Verification items for the finished model (mm, model axes). A direction names the side the tool comes from. Round coordinates to 2 decimals unless told otherwise and drop trailing zeros. Order: outer loops, then holes, each group sorted by start corner. A loop starts at its lowest first (then second) coordinate and runs counter-clockwise, first axis right, second up. Notation, with made-up numbers: (-6, 21.25) -> (31, 21.25) arc R16 cw to (31, 46.25) -> close; hole circle Ø9 at (15.5, 60.25). An arc over 180 degrees is marked (long way). Return JSON: item names as keys, results as strings. Group by question number.
1) Draft check along Y on faces 1 (the cylindrical face through (-48.007, -16.606, 4.93)), 2 (the cylindrical face through (48.007, 16.606, 4.93)), 3 (the cylindrical face through (-48.953, 2.154, 24.157)), 4 (the flat face through (0, 12.5, 15)). Enter one of: pulls with the +Y half, pulls with the -Y half, needs draft (parallel to the pull), parting line crosses it, or undercut.
2) Section check B-B on x = -28. Enter the section's corners in (y, z).
3) Section check C-C on z = 32.5. Enter the section's corners in (x, y).
4) Section check D-D on x = 33. Enter the section's corners in (y, z), plus the area to 3 significant figures.
5) Tool access check on faces 5 (the flat face through (15, -59, 5)), 6 (the flat face through (-59, 15, 5)), 7 (the flat face through (-7, 10, 15)). Record the directions out of +Z, -Z, +X, -X, +Y, -Y that give a thin tool (end or side, any length) a straight path to the whole face; none if there is none.
6) Depth check by flat-ended pin: pin 1 (0.7 mm diameter, centred on x = 5, z = 14, fed in from +Y); pin 2 (8 mm diameter, centred on x = 61.5, z = 4.5, fed in from +Y); pin 3 (11 mm diameter, centred on y = -60, z = 3, fed in from +X); pin 4 (12 mm diameter, centred on x = 35.5, y = -9, fed in from -Z). Enter the tip coordinate at first touch or a pass-through.
7) Section check A-A on y = 32. Enter the section's corners in (x, z), plus the area to 3 significant figures.
8) Scan lines: L1, parallel to X at y = 60, z = 2.5; L2, parallel to X at y = 14, z = 23. Record each from-to range of solid material in increasing order.
```python
from build123d import *

# Parameters (mm, degrees)
SZKIC1_R                    = 49
SZKIC1_R_2                  = 44
DODANIE_WYCI_GNI_CIE1_DEPTH = 49
DODANIE_WYCI_GNI_CIE2_DEPTH = 30
SZKIC3_W                    = 21
SZKIC3_H                    = 41
WYTNIJ_WYCI_GNI_CIE1_DEPTH  = 30
WYTNIJ_WYCI_GNI_CIE2_DEPTH  = 20
OTW_R_POD_RUB_M21_D         = 2.6
WYTNIJ_WYCI_GNI_CIE3_REACH  = 77.512
SZKIC8_W                    = 7
SZKIC8_H                    = 5
DODANIE_WYCI_GNI_CIE3_DEPTH = 10
OTW_R_POD_RUB_M22_D         = 2.6
SZYK_KO_OWY1_COUNT          = 4
ZAOKR_GLENIE1_R             = 10


with BuildPart() as part:
    # Szkic1 → Dodanie-wyciągnięcie1 (new body)
    with BuildSketch(Plane.XY):
        Circle(SZKIC1_R)
        Circle(SZKIC1_R_2, mode=Mode.SUBTRACT)
    extrude(amount=DODANIE_WYCI_GNI_CIE1_DEPTH)

    # Szkic2 → Dodanie-wyciągnięcie2 (add)
    with BuildSketch(Plane.XY):
        with BuildLine():
            Line((15, 46.647615159), (15, -46.647615159))
            ThreePointArc((15, -46.647615159), (0, -49), (-15, -46.647615159))
            Line((-15, -46.647615159), (-15, 46.647615159))
            ThreePointArc((-15, 46.647615159), (0, 49), (15, 46.647615159))
        make_face()
    extrude(amount=DODANIE_WYCI_GNI_CIE2_DEPTH)

    # Szkic3 → Wytnij-wyciągnięcie1 (cut)
    with BuildSketch(Plane.XY.offset(30)):
        with Locations((0, -10.5)):
            Rectangle(SZKIC3_W, SZKIC3_H)
    extrude(amount=-WYTNIJ_WYCI_GNI_CIE1_DEPTH, mode=Mode.SUBTRACT)

    # Szkic5 → Wytnij-wyciągnięcie2 (cut)
    with BuildSketch(Plane(origin=(0, 0, 0), x_dir=(-1, 0, 0), z_dir=(0, 0, -1))):
        Polygon((6.154700538, -33), (3.845299462, -33), (2.690598923, -35), (3.845299462, -37), (6.154700538, -37), (7.309401077, -35), align=None)
    wytnij_wyci_gni_cie2 = extrude(amount=-WYTNIJ_WYCI_GNI_CIE2_DEPTH, mode=Mode.SUBTRACT)

    # Szkic-szyk1: Wytnij-wyciągnięcie2 at 3 more places
    with Locations((0, 49.5, 0), (10, 49.5, 0), (10, 0, 0)):
        add(wytnij_wyci_gni_cie2, mode=Mode.SUBTRACT)

    # Otwór pod śrubę M21 (through all)
    with Locations(Plane(origin=(0, 0, 20), x_dir=(-1, 0, 0), z_dir=(0, 0, -1))):
        with Locations((-5, 14.5)):
            otw_r_pod_rub_m21 = Hole(OTW_R_POD_RUB_M21_D / 2)

    # Szkic-szyk2: Otwór pod śrubę M21 at 3 more places
    with Locations((-10, 0, 0), (0, -49.5, 0), (-10, -49.5, 0)):
        add(otw_r_pod_rub_m21, mode=Mode.SUBTRACT)

    # Szkic8 → Wytnij-wyciągnięcie3 (cut, up to next)
    with BuildSketch(Plane.XY.offset(30), mode=Mode.PRIVATE) as wytnij_wyci_gni_cie3_sk1:
        with Locations((0, 10)):
            Rectangle(SZKIC8_W, SZKIC8_H)
    wytnij_wyci_gni_cie3_tool1 = extrude(wytnij_wyci_gni_cie3_sk1.sketch, amount=-WYTNIJ_WYCI_GNI_CIE3_REACH, mode=Mode.PRIVATE) & part.part
    add(wytnij_wyci_gni_cie3_tool1.solids().sort_by_distance((0, 10, 30))[0], mode=Mode.SUBTRACT)

    # Szkic9 → Dodanie-wyciągnięcie3 (add)
    with BuildSketch(Plane(origin=(0, 0, 0), x_dir=(-1, 0, 0), z_dir=(0, 0, -1))):
        with BuildLine():
            Line((-75, -15), (-41.36423576, -15))
            ThreePointArc((-41.36423576, -15), (-44, 0), (-41.36423576, 15))
            Line((-41.36423576, 15), (-75, 15))
            Line((-75, 15), (-75, -15))
        make_face()
    dodanie_wyci_gni_cie3 = extrude(amount=-DODANIE_WYCI_GNI_CIE3_DEPTH)

    # Otwór pod śrubę M22 (through all)
    with Locations(Plane.XY.offset(10)):
        with Locations((60, 0)):
            otw_r_pod_rub_m22 = Hole(OTW_R_POD_RUB_M22_D / 2)

    # Szyk kołowy1: Dodanie-wyciągnięcie3, Otwór pod śrubę M22 ×4 about axis
    szyk_ko_owy1_axis = Axis((0, 0, 0), (0, 0, 1))
    add([dodanie_wyci_gni_cie3.rotate(szyk_ko_owy1_axis, i * 360 / SZYK_KO_OWY1_COUNT) for i in range(1, SZYK_KO_OWY1_COUNT)])
    add([otw_r_pod_rub_m22.rotate(szyk_ko_owy1_axis, i * 360 / SZYK_KO_OWY1_COUNT) for i in range(1, SZYK_KO_OWY1_COUNT)], mode=Mode.SUBTRACT)

    # Zaokrąglenie1
    zaokr_glenie1_edges = [part.edges().sort_by_distance(p)[0] for p in [
        (46.647615159, -15, 5),
        (46.647615159, 15, 5),
        (75, 15, 5),
        (75, -15, 5),
        (15, -46.647615159, 5),
        (15, -75, 5),
        (-15, -75, 5),
        (-15, -46.647615159, 5),
        (-46.647615159, -15, 5),
        (-75, -15, 5),
        (-75, 15, 5),
        (-46.647615159, 15, 5),
        (-15, 46.647615159, 5),
        (-15, 75, 5),
        (15, 75, 5),
        (15, 46.647615159, 5),
    ]]
    fillet(zaokr_glenie1_edges, radius=ZAOKR_GLENIE1_R)


solid = part.part
```
Check result:
{
 "1": {"face 1": "pulls with the -Y half", "face 2": "pulls with the +Y half", "face 3": "parting line crosses it", "face 4": "undercut"},
 "2": {"outline": "(-40.21, 0) -> (-33.94, 0) -> (-33.94, 49) -> (-40.21, 49) -> close; (33.94, 0) -> (40.21, 0) -> (40.21, 49) -> (33.94, 49) -> close"},
 "3": {"outline": "circle Ø98 at (0, 0); hole circle Ø88 at (0, 0)"},
 "4": {"outline": "(-36.22, 0) -> (-29.1, 0) -> (-29.1, 49) -> (-36.22, 49) -> close; (29.1, 0) -> (36.22, 0) -> (36.22, 49) -> (29.1, 49) -> close", "area": "698 mm^2"},
 "5": {"face 5": "+Z, -Z, +X, -Y", "face 6": "+Z, -Z, -X, +Y", "face 7": "+Z, -Z"},
 "6": {"pin 1": "y = 48.78", "pin 2": "y = 15", "pin 3": "x = 15", "pin 4": "through"},
 "7": {"outline": "(-37.11, 0) -> (-30.2, 0) -> (-30.2, 49) -> (-37.11, 49) -> close; (-15, 0) -> (15, 0) -> (15, 30) -> (-15, 30) -> close; (30.2, 0) -> (37.11, 0) -> (37.11, 49) -> (30.2, 49) -> close", "area": "1,580 mm^2"},
 "8": {"L1": "-15 to -1.3, 1.3 to 15", "L2": "-46.96 to -41.71, -15 to -6.2, -3.8 to 3.8, 6.2 to 15, 41.71 to 46.96"}
}
